Verification items for this drawing (mm, ordinates from the low corner). Coordinates: 2 decimals unless noted, no trailing zeros. Order: outer loops, then holes, each group sorted by start corner. A loop starts at its lowest first (then second) coordinate and runs counter-clockwise, first axis right, second up. Notation, with made-up numbers: (64.25, 69) -> (86.25, 69) arc R15 cw to (86.25, 86) -> close; hole circle Ø2 at (81.25, 56). An arc over 180 degrees is marked (long way). Answer in a Markdown table with one row per item. Add a question column.
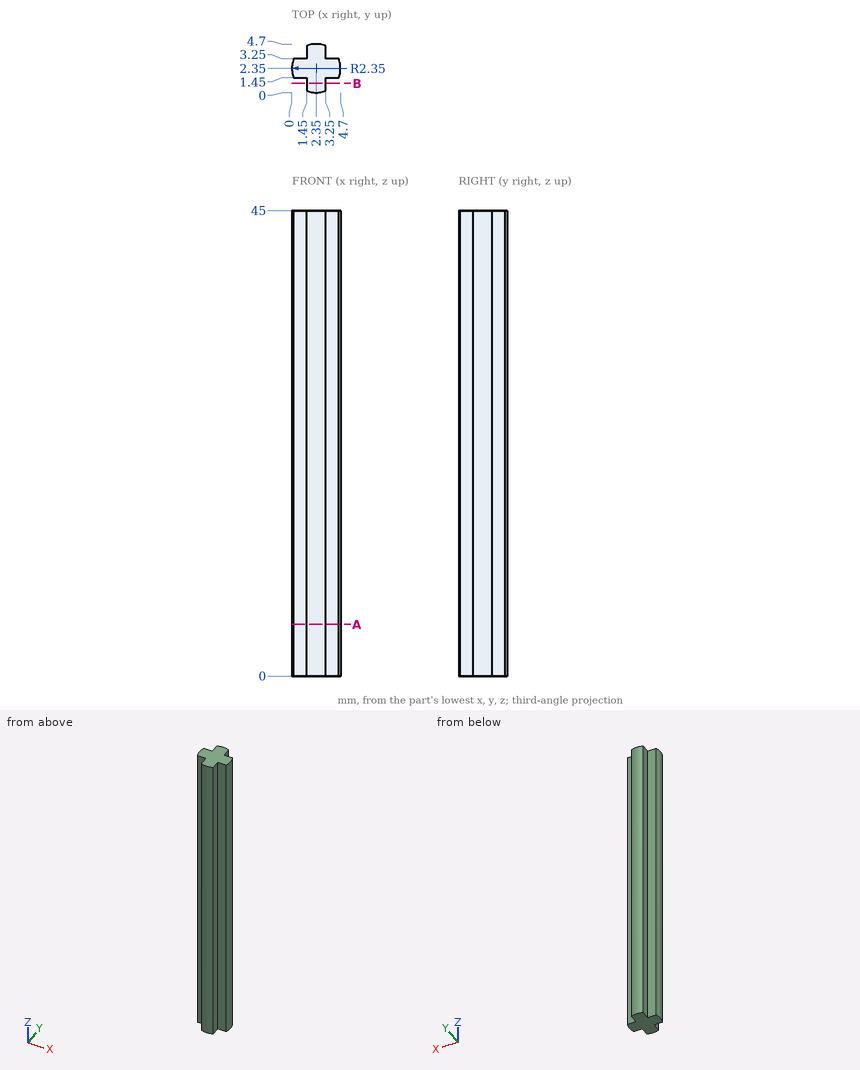
(1) Cross-section at A-A (z = 5). Enter the section's corners in (x, y), plus the area to 3 significant figures.
(2) Go/stop test with flat-tipped pins: P1, Ø1.4, axis at x = 1, z = 15, coming from the -Y side; P2, Ø1.4, axis at y = 4, z = 33.5, coming from the -X side; P3, Ø0.6, axis at x = 3.5, z = 24.5, coming from the +Y side; P4, Ø2, axis at x = 2, z = 35.5, coming from the +Y side. Record where each tip stops, or that it passes through.
(3) Cross-section at B-B (y = 0.9). Enter the section's corners in (x, z).
(4) Scan lines: line 1 along Y through (x, z) = (1, 23); line 2 along Y through (x, z) = (2.2, 9.5). Record each from-to range of solid material in increasing order.
Checks:
| question | item | result |
|---|---|---|
| 1 | outline | (0.18, 1.45) -> (1.45, 1.45) -> (1.45, 0.18) arc R2.35 ccw to (3.25, 0.18) -> (3.25, 1.45) -> (4.52, 1.45) arc R2.35 ccw to (4.52, 3.25) -> (3.25, 3.25) -> (3.25, 4.52) arc R2.35 ccw to (1.45, 4.52) -> (1.45, 3.25) -> (0.18, 3.25) arc R2.35 ccw to start |
| 1 | area | 13.3 mm² |
| 2 | P1 | y = 0.09 |
| 2 | P2 | x = 1.45 |
| 2 | P3 | y = 4.54 |
| 2 | P4 | y = 4.7 |
| 3 | outline | (1.45, 0) -> (3.25, 0) -> (3.25, 45) -> (1.45, 45) -> close |
| 4 | line 1 | 1.45 to 3.25 |
| 4 | line 2 | 0 to 4.7 |
